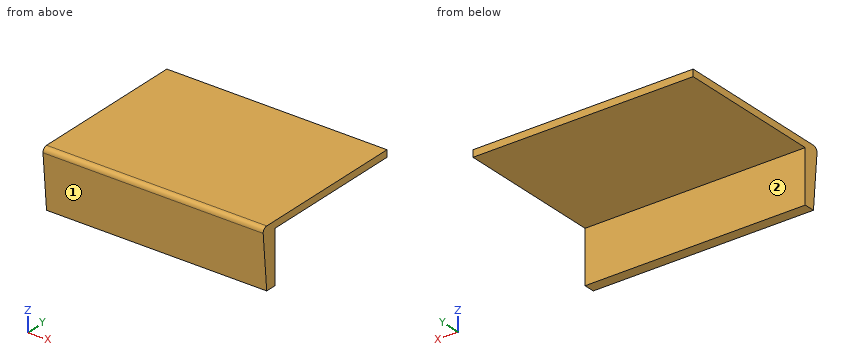
```python
from build123d import *

# Parameters (mm, degrees)
F1_DEPTH = 609.6


with BuildPart() as f1:
    # F0 (on Right) → F1 (new body)
    with BuildSketch(Plane.YZ):
        with BuildLine():
            Line((-143.804814, -89.440058), (-143.804814, 55.022442))
            Line((-143.804814, 55.022442), (264.182686, 55.022442))
            Line((264.182686, 55.022442), (264.182686, 74.072442))
            Line((264.182686, 74.072442), (-173.666681, 74.072442))
            ThreePointArc((-173.666681, 74.072442), (-183.036482, 70.278105), (-186.667314, 60.843743))
            Line((-186.667314, 60.843743), (-173.74242, -89.440058))
            Line((-173.74242, -89.440058), (-143.804814, -89.440058))
        make_face()
    extrude(amount=F1_DEPTH)


solid = f1.part
```
Model file for the job. Use its own axes, mm. Face numbers are marked on the shaded views. A direction names the side the tool comes from. Coordinates: 2 decimals unless noted, no trailing zeros. Loops run counter-clockwise (first coordinate to the right, second up) from the corner with the lowest first, then second, coordinate; pieces in that order, holes last. Notation, with made-up numbers: (2, 47.25) - (9, 47.25) arc R28 cw to (9, 83.25) - close; hole circle Ø9 at (11.5, -33). An arc over 180 degrees is marked (long way). Write item = value, one per line. Start each with the question number.
Item 1: Saw through at A-A, the plane x = 521.5. List the corners of the cut face in (y, z).
Item 2: Saw through at C-C, the plane z = -23. List the corners of the cut face in (x, y), then the cut area to 3 significant figures.
Item 3: Saw through at B-B, the plane y = -72. List the corners of the cut face in (x, z), then the cut area to 3 significant figures.
Item 4: Wall check: probe 1 along Z at (x, y) = (521, -71); probe 2 along Z at (x, y) = (449.5, -164.5); probe 3 along Y at (x, z) = (366.5, 34.5). Give the ranges that are in metal, low to high. Write a range as [from, to].
Item 5: 3-axis set-ups, long thin cutter, end or side, ignore diameter. For the marked faces 1 and 2: which of +Z, -Z, +X, -X, +Y, -Y reach the whole face in a straight line?
Item 6: Drop flat-ended pins along their axis: pin 1 Ø4 at (x, z) = (518, 44.5) entering from -Y; pin 2 Ø1 at (x, z) = (235, 24.5) entering from +Y; pin 3 Ø1 at (x, y) = (340.5, -93.5) entering from -Z. Give the stop position or say it passes through.
Answers:
q1.outline = (-186.67, 60.84) - (-173.74, -89.44) - (-143.8, -89.44) - (-143.8, 55.02) - (264.18, 55.02) - (264.18, 74.07) - (-173.67, 74.07) arc R12.7 ccw to start
q2.outline = (0, -179.46) - (609.6, -179.46) - (609.6, -143.8) - (0, -143.8) - close
q2.area = 21,700 mm2
q3.outline = (0, 55.02) - (609.6, 55.02) - (609.6, 74.07) - (0, 74.07) - close
q3.area = 11,600 mm2
q4.probe_1 = [55.02, 74.07]
q4.probe_2 = [-89.44, 74.07]
q4.probe_3 = [-184.4, -143.8]
q5.face_1 = -Z, +X, -X, -Y
q5.face_2 = -Z, +X, -X, +Y
q6.pin_1 = -185.43
q6.pin_2 = -143.8
q6.pin_3 = 55.02
